from build123d import *

# Parameters (mm, degrees)
SKETCH1_W                = 88
SKETCH1_H                = 95
BOSS_EXTRUDE1_DEPTH      = 3
BOSS_EXTRUDE2_DEPTH      = 40
BOSS_EXTRUDE2_DEPTH_BACK = 1
SKETCH2_W                = 88
SKETCH2_H                = 3
SKETCH3_R                = 15
CUT_EXTRUDE1_DEPTH       = 10
FILLET1_R                = 3
FILLET2_R                = 2
SKETCH5_R                = 3.935
CUT_EXTRUDE3_DEPTH       = 10
LPATTERN1_COUNT          = 2
LPATTERN1_PITCH          = 20
FILLET3_R                = 2
SKETCH6_R                = 3.325
CUT_EXTRUDE4_DEPTH       = 10
CIRPATTERN1_COUNT        = 6


with BuildPart() as part:
    # Sketch1 → Boss-Extrude1 (new body)
    with BuildSketch(Plane.XY):
        Rectangle(SKETCH1_W, SKETCH1_H)
    extrude(amount=BOSS_EXTRUDE1_DEPTH)

    # Sketch2 → Boss-Extrude2 (add, two sides: drawn at the far end of the back side and taken through both)
    with BuildSketch(Plane.XY.offset(3).offset(-BOSS_EXTRUDE2_DEPTH_BACK)):
        with Locations((0, 46)):
            Rectangle(SKETCH2_W, SKETCH2_H)
    extrude(amount=BOSS_EXTRUDE2_DEPTH + BOSS_EXTRUDE2_DEPTH_BACK)

    # Sketch3 → Cut-Extrude1 (cut)
    with BuildSketch(Plane(origin=(0, 0, 0), x_dir=(-1, 0, 0), z_dir=(0, 0, -1))):
        Circle(SKETCH3_R)
    extrude(amount=-CUT_EXTRUDE1_DEPTH, mode=Mode.SUBTRACT)

    # Fillet1
    fillet1_edges = [part.edges().sort_by_distance(p)[0] for p in [
        (0, 47.5, 0),
    ]]
    fillet(fillet1_edges, radius=FILLET1_R)

    # Fillet2
    fillet2_edges = [part.edges().sort_by_distance(p)[0] for p in [
        (0, 44.5, 3),
    ]]
    fillet(fillet2_edges, radius=FILLET2_R)

    # Sketch5 → Cut-Extrude3 (cut)
    with BuildSketch(Plane(origin=(0, 47.5, 0), x_dir=(1, 0, 0), z_dir=(0, 1, 0))):
        with Locations(Location((0, -13, 0), (0, 0, 270))):
            Circle(SKETCH5_R)
    cut_extrude3 = extrude(amount=-CUT_EXTRUDE3_DEPTH, mode=Mode.SUBTRACT)

    # LPattern1: Cut-Extrude3 ×2
    with Locations(*[(0, 0, i * LPATTERN1_PITCH) for i in range(1, LPATTERN1_COUNT)]):
        add(cut_extrude3, mode=Mode.SUBTRACT)

    # Fillet3
    fillet3_edges = [part.edges().sort_by_distance(p)[0] for p in [
        (-44, 46, 43),
        (44, 46, 43),
        (44, -47.5, 1.5),
        (-44, -47.5, 1.5),
    ]]
    fillet(fillet3_edges, radius=FILLET3_R)

    # Sketch6 → Cut-Extrude4 (cut)
    with BuildSketch(Plane.XY.offset(3)):
        with Locations((35, 0)):
            Circle(SKETCH6_R)
    cut_extrude4 = extrude(amount=-CUT_EXTRUDE4_DEPTH, mode=Mode.SUBTRACT)

    # CirPattern1: Cut-Extrude4 ×6 about axis
    cirpattern1_axis = Axis((0, 0, 0), (0, 0, 1))
    for i in range(1, CIRPATTERN1_COUNT):
        add(cut_extrude4.rotate(cirpattern1_axis, i * 360 / CIRPATTERN1_COUNT), mode=Mode.SUBTRACT)


solid = part.part
Build history of the part. All positions in model axes, mm. A direction names the side the tool comes from. Round coordinates to 2 decimals unless told otherwise and drop trailing zeros. Write each loop counter-clockwise with the first axis right and the second up, starting at its lowest first coordinate (ties: lowest second). Pieces come first, ordered by that corner, then holes. Notation, with made-up numbers: M -23.5,54 L -13.5,54 A19 ccw -13.5,83 Z; hole C -14.5,24.25 d2. An arc over 180 degrees is marked long. Answer as a JSON object with one key per item and string values. Group by question number.
(1) Drill centre lines: L1, parallel to Y at x = 17, z = 1; L2, parallel to X at y = 46.5, z = 33 (3 decimals); L3, parallel to Y at x = 17.5, z = 1.8. Where is each one in solid material? Low to high.
(2) Cut at C-C (x = 17.5). Give the cut face in (y, z), and give its area (3 significant figures).
(3) Cut at A-A (z = 33). Give the cut face in (x, y) (3 decimals), and give its area (3 significant figures).
(4) Flat gauge pins, fed straight in: pin 1 (10 mm diameter, centred on x = 0, z = 33, fed in from -Y); pin 2 (8 mm diameter, centred on x = -17, y = 2, fed in from +Z). Where does each tip first touch, or does it go through?
(5) Cut at D-D (y = 6). Give the cut face in (x, z), and give its area (3 significant figures).
(6) Which spindle directions (+Z, -Z, +X, -X, +Y, -Y) get a long thin tool onto all of the face, cutting with end or side? Do faces 4 (the flat face through (-10, -12, 3)), 5 (the cylindrical face through (17.933, -33.608, 1.521)). Say none if no direction does.
(7) Cut at B-B (x = 35). Give the cut face in (y, z) (3 decimals).
(8) Mould opens along Y. For faces 1 (the cylindrical face through (1.182, 46.021, 16.753)), 2 (the cylindrical face through (-15.71, -27.51, 1.52)), 3 (the flat face through (-1, 47.5, 23)) say: pulls with the +Y half, pulls with the -Y half, needs draft (parallel to the pull), parting line crosses it, or undercut.
Responses:
{
 "1": {"L1": "y = -47.5 to -33.6, -27.02 to 27.02, 33.6 to 46.74", "L2": "x = -44 to -3.935, 3.935 to 44", "L3": "y = -47.5 to -33.64, -26.99 to 26.99, 33.64 to 47.25"},
 "2": {"outline": "M -47.5,0 L -33.64,0 L -33.64,3 L -47.5,3 Z; M -26.99,0 L 26.99,0 L 26.99,3 L -26.99,3 Z; M 33.64,0 L 44.5,0 A3 ccw 47.5,3 L 47.5,43 L 44.5,43 L 44.5,5 A2 cw 42.5,3 L 33.64,3 Z", "area": "364 mm2"},
 "3": {"outline": "M -44,44.5 L -3.935,44.5 L -3.935,47.5 L -44,47.5 Z; M 3.935,44.5 L 44,44.5 L 44,47.5 L 3.935,47.5 Z", "area": "240 mm2"},
 "4": {"pin 1": "stops at y = 44.5", "pin 2": "stops at z = 3"},
 "5": {"outline": "M -44,0 L -13.75,0 L -13.75,3 L -44,3 Z; M 13.75,0 L 44,0 L 44,3 L 13.75,3 Z", "area": "182 mm2"},
 "6": {"face 4": "+Z, +X, -X, -Y", "face 5": "+Z, -Z"},
 "7": {"outline": "M -47.5,0 L -3.325,0 L -3.325,3 L -47.5,3 Z; M 3.325,0 L 44.5,0 A3 ccw 47.5,3 L 47.5,43 L 44.5,43 L 44.5,5 A2 cw 42.5,3 L 3.325,3 Z"},
 "8": {"face 1": "needs draft", "face 2": "undercut", "face 3": "pulls with the +Y half"}
}
